The listing builds one solid part. Answer for the finished solid, in the listing's coordinates (mm). Face numbers are marked on the shaded views. A direction names the side the tool comes from. Give positions to 0.01 mm unless a question says otherwise; leave off trailing zeros. Write each loop counter-clockwise with the first axis right and the second up, starting at its lowest first coordinate (ties: lowest second). Pieces come first, ordered by that corner, then holes. Notation, with made-up numbers: M 12,55 L 44,55 A15 ccw 44,79 Z; hole C -17,56 d9. An arc over 180 degrees is marked long. Return JSON: item names as keys, results as strings.
from build123d import *

# Parameters (mm, degrees)
F0_R        = 2.5
F1_DEPTH    = 20
F3_DEPTH    = 16
F4_T2_ANGLE = 304.0474034012
F4_T4_ANGLE = 123.8663608487
F5_SIZE     = 0.49999


# Not quite as in the source:
# - a fillet or chamfer that OpenCascade refuses, or shapes differently, is made with other operations: its cross-section is extruded or revolved along the edge and cut away or added
# - a fillet or chamfer is up to 0.001 mm smaller than in the source, because OpenCascade refuses the exact size


with BuildPart() as f1:
    # F0 (on Top) → F1 (new body)
    with BuildSketch(Plane.XY):
        Circle(F0_R)
    extrude(amount=F1_DEPTH)

    # F2 (on face) → F3 (cut)
    with BuildSketch(Plane.XY.offset(20)):
        with BuildLine():
            ThreePointArc((1.5, 2), (0, 2.5), (-1.5, 2))
            Line((-1.5, 2), (1.5, 2))
        make_face()
    extrude(amount=-F3_DEPTH, mode=Mode.SUBTRACT)

    # F4: chamfer of 0.5 on 1 edges, made by hand

    # F4_s1 → F4_t2 (revolve, cut)
    with BuildSketch(Plane(origin=(0, 0, 0), x_dir=(0, 0, 1), z_dir=(0.8285746432, -0.5598786125, 0))):
        with BuildLine():
            Line((19.4858578644, -2.5141421356), (20.0141421356, -1.9858578644))
            Line((20.0141421356, -1.9858578644), (20.0241421356, -1.9858578644))
            ThreePointArc((20.0241421356, -1.9858578644), (20.01, -2.2429289322), (20.01, -2.5))
            Line((20.01, -2.5), (20, -2.51))
            ThreePointArc((20, -2.51), (19.7429289322, -2.51), (19.4858578644, -2.5241421356))
            Line((19.4858578644, -2.5241421356), (19.4858578644, -2.5141421356))
        make_face()
    revolve(axis=Axis((0, 0, 20), (0, 0, 1)), revolution_arc=F4_T2_ANGLE, mode=Mode.SUBTRACT)

    # F4_s3 → F4_t4 (revolve, cut)
    with BuildSketch(Plane.XZ):
        with BuildLine():
            Line((2.5141421356, 19.4858578644), (1.9858578644, 20.0141421356))
            Line((1.9858578644, 20.0141421356), (1.9858578644, 20.0241421356))
            ThreePointArc((1.9858578644, 20.0241421356), (2.2429289322, 20.01), (2.5, 20.01))
            Line((2.5, 20.01), (2.51, 20))
            ThreePointArc((2.51, 20), (2.51, 19.7429289322), (2.5241421356, 19.4858578644))
            Line((2.5241421356, 19.4858578644), (2.5141421356, 19.4858578644))
        make_face()
    revolve(axis=Axis((0, 0, 20), (0, 0, 1)), revolution_arc=F4_T4_ANGLE, mode=Mode.SUBTRACT)

    # F5 (size 0.5 in the source; OpenCascade refuses exactly that, so slightly less here)
    f5_edges = [f1.edges().sort_by_distance(p)[0] for p in [
        (0, 2, 4),
    ]]
    chamfer(f5_edges, length=F5_SIZE)


solid = f1.part
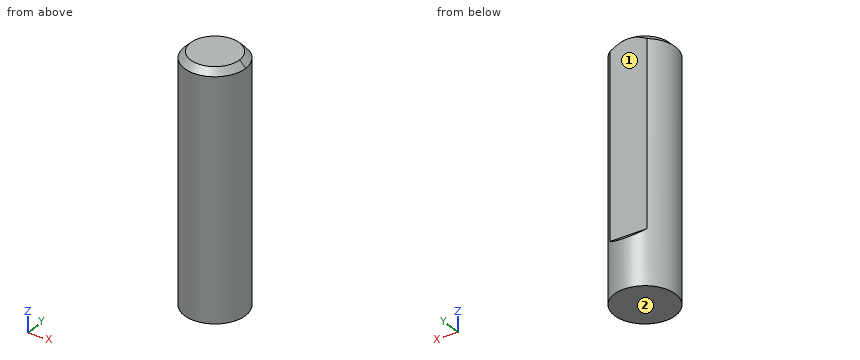
Item 1: A cutting plane is placed at A-A, the plane z = 18.25. Write down the section's boundary in (x, y).
Geometry results:
{"outline": "M -1.5,2 A2.5 ccw long 1.5,2 Z"}
Item 2: Given pin 1 Ø1.5 at (x, z) = (0.5, 10.5) entering from +Y; pin 2 Ø1 at (y, z) = (1, 5.5) entering from +X; pin 3 Ø2 at (x, z) = (-1, 4.5) entering from +Y, each flat-ended and moving along its own axis, determine where each tip first touches the part or whether it passes through.
Geometry results:
{"pin 1": "stops at y = 2", "pin 2": "stops at x = 2.45", "pin 3": "stops at y = 2.5"}
Item 3: Which of the six approach directions +Z, -Z, +X, -X, +Y, -Y give full straight-line access (tool end or side, diameter ignored) to the marked faces 1 and 2?
Geometry results:
{"face 1": "+Z, +X, -X, +Y", "face 2": "-Z, +X, -X, +Y, -Y"}
Item 4: A cutting plane is placed at B-B, the plane z = 3.5. Write down the section's boundary in (x, y).
Geometry results:
{"outline": "C 0,0 d5"}
Item 5: Find the intervals of material crossed by line 1 (X direction, y = -0.1, z = 17.25); line 2 (Y direction, x = -0.05, z = 12.75); line 3 (X direction, y = -2, z = 1.25), in increasing order.
Geometry results:
{"line 1": "x = -2.5 to 2.5", "line 2": "y = -2.5 to 2", "line 3": "x = -1.5 to 1.5"}
